Read the model definition and answer for the solid it produces. Units are mm, in the model's axes. A direction names the side the tool comes from. Give positions to 0.01 mm unless a question says otherwise; leave off trailing zeros. Loops run counter-clockwise (first coordinate to the right, second up) from the corner with the lowest first, then second, coordinate; pieces in that order, holes last. Notation, with made-up numbers: (0, 70.25) - (41, 70.25) arc R18 ccw to (41, 83.25) - close; hole circle Ø5 at (-2.5, 65). An arc over 180 degrees is marked (long way). Write each question's results on one line, items separated by ' | '. Start each with the question number.
Q1. Find the intervals of material crossed by line 1 (Z direction, x = 65, y = 6) (3 decimals); line 2 (Z direction, x = -13.5, y = 45) (3 decimals); line 3 (Y direction, x = 1, z = 20.5), in increasing order. Write a range as from..to.
Q2. The part is cut by section B-B, the plane y = -30. Write down the section's boundary in (x, z) (3 decimals), plus the area to 3 significant figures.
Q3. Determine the mould class of faces 1 (the cylindrical face through (46.301, -0.356, 37.575)), 2 (the cylindrical face through (30.3, -16.79, 48.21)), 3 (the flat face through (-1, -63.5, 0)) for opening direction Z: +Z half, -Z half, draft (parallel to the pull), parting line (faces both ways), or undercut.
Q4. The part is cut by section A-A, the plane z = -4.5. Write down the section's boundary in (x, y) (3 decimals), plus the area to 3 significant figures.
Q5. Given pin 1 (12 mm diameter, centred on x = 40, z = 22, fed in from -Y); pin 2 (12 mm diameter, centred on y = 32, z = 53, fed in from -X); pin 3 (2 mm diameter, centred on y = 2.5, z = 45, fed in from -X); pin 4 (3 mm diameter, centred on y = -26, z = 10, fed in from +X) (3 decimals), each flat-ended and moving along its own axis, determine where each tip first touches the part or whether it passes through.
Q6. For faces 4 (the flat face through (-5, 7.938, 30)), 5 (the flat face through (22.225, -17, 17)), 6 (the flat face through (41.275, -1, 4)), determine the directions among +Z, -Z, +X, -X, +Y, -Y from which every point of the face is accessible in a straight line to the end or side of a thin tool.
```python
from build123d import *

# Parameters (mm, degrees)
F1_DEPTH = 63.5
F0_W     = 25.4
F0_H     = 19.05
F0_H_2   = 4.7752
F0_H_3   = 4.7498
F2_DEPTH = 25.4
F3_DEPTH = 7.9375


with BuildPart() as f1:
    # F0 (on Front) → F1 (new body, symmetric)
    with BuildSketch(Plane.XZ):
        Polygon((22.225, 9.525), (-41.275, 9.525), (-41.275, -9.525), (41.275, -9.525), (41.275, 9.525), align=None)
    extrude(amount=F1_DEPTH, both=True)

    # F0 (on Front) → F2 (join, symmetric)
    with BuildSketch(Plane.XZ):
        with BuildLine():
            Line((22.225, 25.2490305709), (22.225, 9.525))
            Line((22.225, 9.525), (41.275, 9.525))
            Line((41.275, 9.525), (41.275, 25.2490305709))
            ThreePointArc((41.275, 25.2490305709), (46.4375854994, 37.7126145006), (58.9011694291, 42.8752))
            Line((58.9011694291, 42.8752), (60.325, 42.8752))
            Line((60.325, 42.8752), (60.325, 61.9252))
            Line((60.325, 61.9252), (58.9011694291, 61.9252))
            add(Edge.make_bspline(
                [(50.3021553642, 60.9028993807), (53.2386856035, 61.3461922801), (56.1133148393, 61.6898187514), (58.9011694291, 61.9252)],
                knots=[105.260953705, 105.260953705, 105.260953705, 105.260953705, 113.0532877962, 113.0532877962, 113.0532877962, 113.0532877962], degree=3))
            ThreePointArc((50.3021553642, 60.9028993807), (30.0869342253, 47.9400255604), (22.225, 25.2490305709))
        make_face()
        with Locations((73.025, 52.4002)):
            Rectangle(F0_W, F0_H)
        with Locations((73.025, 40.4876)):
            Rectangle(F0_W, F0_H_2)
        with Locations((73.025, 64.3001)):
            Rectangle(F0_W, F0_H_3)
        Polygon((85.725, 66.675), (85.725, 61.9252), (85.725, 42.8752), (85.725, 38.1), (111.125, 38.1), (111.125, 66.675), align=None)
    extrude(amount=F2_DEPTH, both=True)

    # F0 (on Front) → F3 (join, symmetric)
    with BuildSketch(Plane.XZ):
        with BuildLine():
            add(Edge.make_bspline(
                [(-41.275, 9.525), (-40.3280161363, 30.740190757), (10.6347117007, 54.914779156), (50.3021553642, 60.9028993807)],
                knots=[0, 0, 0, 0, 105.260953705, 105.260953705, 105.260953705, 105.260953705], degree=3))
            Line((-41.275, 9.525), (22.225, 9.525))
            Line((22.225, 9.525), (22.225, 25.2490305709))
            ThreePointArc((22.225, 25.2490305709), (30.0869342253, 47.9400255604), (50.3021553642, 60.9028993807))
        make_face()
    extrude(amount=F3_DEPTH, both=True)


solid = f1.part
```
Check sheet entries:
1) line 1: z = 38.1..66.675 | line 2: z = -9.525..9.525 | line 3: y = -7.94..7.94
2) outline: (-41.275, -9.525) - (41.275, -9.525) - (41.275, 9.525) - (-41.275, 9.525) - close | area: 1,570 mm^2
3) face 1: -Z half | face 2: +Z half | face 3: draft
4) outline: (-41.275, -63.5) - (41.275, -63.5) - (41.275, 63.5) - (-41.275, 63.5) - close | area: 10,500 mm^2
5) pin 1: stops at y = -25.4 | pin 2: passes through | pin 3: stops at x = -3.89 | pin 4: stops at x = 41.275
6) face 4: +Z, -X, +Y | face 5: +Z, -X, -Y | face 6: -Z, +X, +Y, -Y
